from build123d import *

# Parameters (mm, degrees)
F0_W     = 50
F0_H     = 10
F1_DEPTH = 25
F2_SIZE  = 4.99999


# Not quite as in the source:
# - a fillet or chamfer is up to 0.001 mm smaller than in the source, because OpenCascade refuses the exact size


with BuildPart() as f1:
    # F0 (on Top) → F1 (new body)
    with BuildSketch(Plane.XY):
        with Locations((-24.5698342215, 0)):
            Rectangle(F0_W, F0_H)
        Polygon((0.4301657785, 5), (0.4301657785, -5), (19.7950825095, 0), align=None)
    extrude(amount=F1_DEPTH)

    # F2 (size 5 in the source; OpenCascade refuses exactly that, so slightly less here)
    f2_edges = [f1.edges().sort_by_distance(p)[0] for p in [
        (-24.569834, -5, 25),
        (-49.569834, 0, 25),
        (-24.569834, 5, 25),
        (10.112624, 2.5, 25),
        (10.112624, -2.5, 25),
    ]]
    chamfer(f2_edges, length=F2_SIZE)


solid = f1.part
Work out the finished part from the listing and answer in its coordinate system (mm). Give positions to 0.01 mm unless a question says otherwise; leave off trailing zeros. Write each loop counter-clockwise with the first axis right and the second up, starting at its lowest first coordinate (ties: lowest second). Pieces come first, ordered by that corner, then holes. Notation, with made-up numbers: M 29,66 L 73,66 A22 cw 73,84 Z; hole C 73.25,84 d8. An arc over 180 degrees is marked long. Answer as CSV lines item,"result".
Q1. Find the intervals of material crossed by probe 1 along Z at (x, y) = (3.5, 2.5); probe 2 along Z at (x, y) = (-30.5, 3.5); probe 3 along Y at (x, z) = (15, 18.25), in increasing order. Write a range as [from, to].
A:
probe 1,"z = [0, 21.65]"
probe 2,"z = [0, 21.5]"
probe 3,"y = [-1.24, 1.24]"
Q2. A cutting plane is placed at C-C on y = -3.5. Write down the section's boundary in (x, z), plus the area to 3 significant figures.
A:
outline,"M -49.57,0 L 6.24,0 L 6.24,20 L 0.24,21.5 L -48.07,21.5 L -49.57,20 Z"
area,"1,190 mm²"
Q3. A cutting plane is placed at B-B on z = 19. Write down the section's boundary in (x, y), plus the area to 3 significant figures.
A:
outline,"M -49.57,-5 L 0.43,-5 L 19.8,0 L 0.43,5 L -49.57,5 Z"
area,"597 mm²"
Q4. A cutting plane is placed at D-D on x = 7. Write down the section's boundary in (y, z).
A:
outline,"M -3.3,0 L 3.3,0 L 3.3,20 L 0,23.2 L -3.3,20 Z"
Q5. Given P1, Ø6, axis at x = 13, z = 17, coming from the +Y side, flat-ended and moving along its own axis, determine where the tip first touches the part or whether it passes through.
A:
P1,"stops at y = 2.53"
